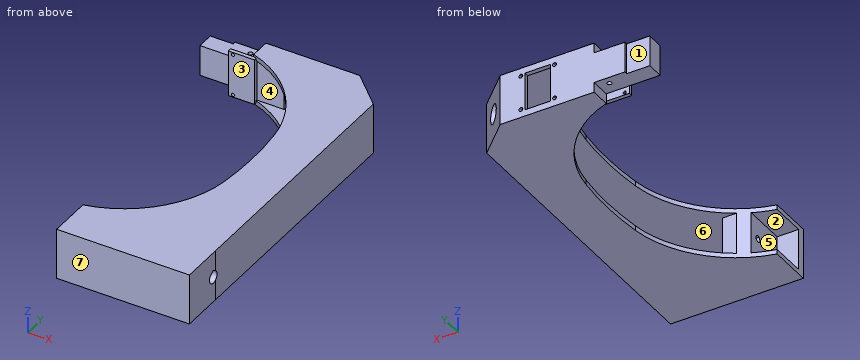
```python
from build123d import *

# Parameters (mm, degrees)
EXTRUDE_6_DEPTH      = 33
CUT_EXTRUDE_START    = 3
CUT_EXTRUDE_2_DEPTH  = 27
EXTRUDE_START        = 6.5
SKETCH_7_W           = 35
SKETCH_7_H           = 13
EXTRUDE_7_DEPTH      = 20
EXTRUDE_START_2      = 1.5
SKETCH_11_W          = 17
SKETCH_11_H          = 2.5
EXTRUDE_15_DEPTH     = 30
CUT_EXTRUDE_START_2  = 180
CUT_EXTRUDE_3_DEPTH  = 10
SKETCH_13_R          = 1.5
CUT_EXTRUDE_4_DEPTH  = 30
SKETCH_14_W          = 15
SKETCH_14_H          = 2
CUT_EXTRUDE_5_DEPTH  = 30
EXTRUDE_START_3      = 11.5
SKETCH_15_W          = 67.299618531
SKETCH_15_H          = 10
EXTRUDE_16_DEPTH     = 10
CUT_EXTRUDE_START_3  = 17
CUT_EXTRUDE_7_DEPTH  = 75
CUT_EXTRUDE_START_4  = 13
CUT_EXTRUDE_9_DEPTH  = 5
SKETCH_20_W          = 16.6
SKETCH_20_H          = 24.7
CUT_EXTRUDE_10_DEPTH = 5
SKETCH_21_R          = 6
CUT_EXTRUDE_11_DEPTH = 5
SKETCH_22_W          = 51
SKETCH_22_H          = 47
CUT_EXTRUDE_12_DEPTH = 27


with BuildPart() as part:
    # Эскиз1 → Бобышка-Вытянуть6 (new body)
    with BuildSketch(Plane.XY):
        with BuildLine():
            Line((4.299618531, 175.402841826), (4.299618531, 188.402841826))
            Line((4.299618531, 188.402841826), (65.299618531, 188.402841826))
            Line((65.299618531, 188.402841826), (86.299618531, 168.402841826))
            Line((86.299618531, 168.402841826), (86.299619, 0))
            Line((86.299619, 0), (86.299619, -28))
            Line((86.299619, -28), (0, -28))
            Line((0, -28), (0, 0))
            ThreePointArc((0, 0), (37.229295141, 21.561020186), (55.173142182, 60.662380285))
            ThreePointArc((55.173142182, 60.662380285), (56.797307883, 87.162380285), (55.173142182, 113.662380285))
            ThreePointArc((55.173142182, 113.662380285), (38.726552267, 151.940422917), (4.299618531, 175.402841826))
        make_face()
    extrude(amount=EXTRUDE_6_DEPTH)

    # Эскиз5 → Вырез-Вытянуть2 (cut)
    with BuildSketch(Plane.XY.offset(CUT_EXTRUDE_START)):
        Polygon((24.099618531, 175.402841826), (4.299618531, 175.402841826), (4.299618531, 169.136823089), (-18.700381469, 169.136823089), (-18.700381469, -23.02337805), (14, -23.02337805), (14, 8.47662195), (81.178938205, 8.47662195), (81.178938205, 169.136823089), (64.099618531, 185.402841826), (24.099618531, 185.402841826), align=None)
    extrude(amount=CUT_EXTRUDE_2_DEPTH, mode=Mode.SUBTRACT)

    # Эскиз7 → Бобышка-Вытянуть7 (add)
    with BuildSketch(Plane.XY.offset(EXTRUDE_START)):
        with Locations((-13.200381469, 181.902841826)):
            Rectangle(SKETCH_7_W, SKETCH_7_H)
    extrude(amount=EXTRUDE_7_DEPTH)

    # Эскиз11 → Бобышка-Вытянуть15 (add)
    with BuildSketch(Plane.XY.offset(EXTRUDE_START_2)):
        with Locations((-2.200381469, 174.152841826)):
            Rectangle(SKETCH_11_W, SKETCH_11_H)
    extrude(amount=EXTRUDE_15_DEPTH)

    # Эскиз12 → Вырез-Вытянуть3 (cut)
    with BuildSketch(Plane(origin=(0, 0, 0), x_dir=(1, 0, 0), z_dir=(0, 1, 0)).offset(CUT_EXTRUDE_START_2)):
        with BuildLine():
            Line((-7.700381469, -31.154700538), (-7.200381469, -30.866025404))
            ThreePointArc((-7.200381469, -30.866025404), (-7.700381469, -29), (-8.200381469, -30.866025404))
            Line((-8.200381469, -30.866025404), (-7.700381469, -31.154700538))
        make_face()
        with BuildLine():
            Line((-7.700381469, -4.154700538), (-7.200381469, -3.866025404))
            ThreePointArc((-7.200381469, -3.866025404), (-7.700381469, -2), (-8.200381469, -3.866025404))
            Line((-8.200381469, -3.866025404), (-7.700381469, -4.154700538))
        make_face()
    extrude(amount=-CUT_EXTRUDE_3_DEPTH, mode=Mode.SUBTRACT)

    # Эскиз13 → Вырез-Вытянуть4 (cut)
    with BuildSketch(Plane.XY):
        with Locations((-2.700381469, 183.402841826)):
            Circle(SKETCH_13_R)
    extrude(amount=CUT_EXTRUDE_4_DEPTH, mode=Mode.SUBTRACT)

    # Эскиз14 → Вырез-Вытянуть5 (cut)
    with BuildSketch(Plane.XY):
        with Locations((-23.200381469, 187.402841826)):
            Rectangle(SKETCH_14_W, SKETCH_14_H)
    extrude(amount=CUT_EXTRUDE_5_DEPTH, mode=Mode.SUBTRACT)

    # Эскиз15 → Бобышка-Вытянуть16 (add)
    with BuildSketch(Plane.XY.offset(EXTRUDE_START_3)):
        with Locations((47.649809735, -2.5)):
            Rectangle(SKETCH_15_W, SKETCH_15_H)
    extrude(amount=EXTRUDE_16_DEPTH)

    # Эскиз17 → Вырез-Вытянуть7 (cut)
    with BuildSketch(Plane(origin=(0, 0, 0), x_dir=(0, 0, -1), z_dir=(1, 0, 0)).offset(CUT_EXTRUDE_START_3)):
        with BuildLine():
            Line((-21.118802154, -2.5), (-19.964101615, -0.5))
            ThreePointArc((-19.964101615, -0.5), (-12.5, -2.5), (-19.964101615, -4.5))
            Line((-19.964101615, -4.5), (-21.118802154, -2.5))
        make_face()
    extrude(amount=CUT_EXTRUDE_7_DEPTH, mode=Mode.SUBTRACT)

    # Эскиз18 → Вырез-Вытянуть9 (cut)
    with BuildSketch(Plane(origin=(0, 0, 0), x_dir=(0, 0, -1), z_dir=(1, 0, 0)).offset(CUT_EXTRUDE_START_4)):
        with BuildLine():
            Line((-18.809401077, -2.5), (-18.232050808, -1.5))
            ThreePointArc((-18.232050808, -1.5), (-14.5, -2.5), (-18.232050808, -3.5))
            Line((-18.232050808, -3.5), (-18.809401077, -2.5))
        make_face()
    extrude(amount=CUT_EXTRUDE_9_DEPTH, mode=Mode.SUBTRACT)

    # Эскиз20 → Вырез-Вытянуть10 (cut)
    with BuildSketch(Plane(origin=(0, 188.402841826, 0), x_dir=(1, 0, 0), z_dir=(0, 1, 0))):
        with Locations((40.95, -16.5)):
            Rectangle(SKETCH_20_W, SKETCH_20_H)
        with BuildLine():
            Line((30, -29.143375673), (30.625, -28.782531755))
            ThreePointArc((30.625, -28.782531755), (30, -26.45), (29.375, -28.782531755))
            Line((29.375, -28.782531755), (30, -29.143375673))
        make_face()
        with BuildLine():
            Line((30, -6.743375673), (30.625, -6.382531755))
            ThreePointArc((30.625, -6.382531755), (30, -4.05), (29.375, -6.382531755))
            Line((29.375, -6.382531755), (30, -6.743375673))
        make_face()
        with BuildLine():
            Line((51.9, -6.743375673), (52.525, -6.382531755))
            ThreePointArc((52.525, -6.382531755), (51.9, -4.05), (51.275, -6.382531755))
            Line((51.275, -6.382531755), (51.9, -6.743375673))
        make_face()
        with BuildLine():
            Line((51.9, -29.143375673), (52.525, -28.782531755))
            ThreePointArc((52.525, -28.782531755), (51.9, -26.45), (51.275, -28.782531755))
            Line((51.275, -28.782531755), (51.9, -29.143375673))
        make_face()
    extrude(amount=-CUT_EXTRUDE_10_DEPTH, mode=Mode.SUBTRACT)

    # Эскиз21 → Вырез-Вытянуть11 (cut)
    with BuildSketch(Plane(origin=(125.147492247, 131.404866859, 0), x_dir=(0, 0, -1), z_dir=(0.689655172, 0.724137931, 0))):
        with Locations((-16.5, 68.147063703)):
            Circle(SKETCH_21_R)
    extrude(amount=-CUT_EXTRUDE_11_DEPTH, mode=Mode.SUBTRACT)

    # Эскиз22 → Вырез-Вытянуть12 (cut)
    with BuildSketch(Plane.XY.offset(CUT_EXTRUDE_START)):
        with Locations((55.799619, -1.5)):
            Rectangle(SKETCH_22_W, SKETCH_22_H)
    extrude(amount=CUT_EXTRUDE_12_DEPTH, mode=Mode.SUBTRACT)


solid = part.part
```
Source: CAD feature listing. Evaluate the final solid. Frame: model axes, mm. Face numbers are marked on the shaded views. A direction names the side the tool comes from. Round coordinates to 2 decimals unless told otherwise and drop trailing zeros. Loops run counter-clockwise (first coordinate to the right, second up) from the corner with the lowest first, then second, coordinate; pieces in that order, holes last.
1. Section query B-B on y = 166. Output: boundary loops of the cut face in (x, z), and give its area (3 significant figures).
2. Section query C-C on y = 58.5. Output: boundary loops of the cut face in (x, z), and give its area (3 significant figures).
3. Access query for the marked faces 1, 2 and 3. Directions: +Z, -Z, +X, -X, +Y, -Y. A direction counts if a zero-diameter tool reaches every point of the face in a straight line with its end or side. Return the directions, or none.
4. Section query A-A on x = 44.5. Output: boundary loops of the cut face in (y, z), and give its area (3 significant figures).
5. Contact query for flat-ended pins moving along their axis: pin 1 (3 mm diameter, centred on y = 41, z = 7.5, fed in from -X); pin 2 (3 mm diameter, centred on y = 180, z = 10, fed in from +X); pin 3 (16 mm diameter, centred on x = -21.5, z = 17.5, fed in from -Y); pin 4 (1.8 mm diameter, centred on x = -7.7, z = 3, fed in from +Y). Output: stop coordinate, or through.
6. Mould query, pull axis X, two halves, no side actions, for the marked faces 4, 5, 6 and 7. Classes: released by +X, released by -X, zero draft, split by the parting line, or undercut.
7. Ray query, L1, parallel to Z at x = 30, y = 187.15; L2, parallel to Z at x = 79.5, y = 120; L3, parallel to Y at x = 9, z = 8. Return the intervals inside material, ascending.
Answers below:
1. outline: (23.37, 0) - (86.3, 0) - (86.3, 33) - (23.37, 33) - (23.37, 30) - (81.18, 30) - (81.18, 3) - (23.37, 3) - close
1. area: 516 mm2
2. outline: (54.87, 0) - (86.3, 0) - (86.3, 33) - (54.87, 33) - (54.87, 30) - (81.18, 30) - (81.18, 3) - (54.87, 3) - close
2. area: 327 mm2
3. face 1: +Z, -Z, -X, +Y
3. face 2: -X
3. face 3: +Z, -Z, -X
4. outline: (-28, 0) - (31.05, 0) - (31.05, 3) - (-25, 3) - (-25, 30) - (31.05, 30) - (31.05, 33) - (-28, 33) - close; (143.9, 0) - (188.4, 0) - (188.4, 4.15) - (185.4, 4.15) - (185.4, 3) - (143.9, 3) - close; (143.9, 30) - (185.4, 30) - (185.4, 28.85) - (188.4, 28.85) - (188.4, 33) - (143.9, 33) - close
4. area: 709 mm2
5. pin 1: stops at x = 81.18
5. pin 2: stops at x = 75.7
5. pin 3: stops at y = 175.4
5. pin 4: passes through
6. face 4: undercut
6. face 5: released by -X
6. face 6: undercut
6. face 7: zero draft
7. L1: z = 0 to 4.05, 6.74 to 26.45, 29.14 to 33
7. L2: z = 0 to 3, 30 to 33
7. L3: y = -28 to -23.02, 175.4 to 188.4
